The model under review builds one solid part; all positions refer to its coordinate system, in mm. A direction names the side the tool comes from. Give positions to 0.01 mm unless a question says otherwise; leave off trailing zeros. Order: outer loops, then holes, each group sorted by start corner. A loop starts at its lowest first (then second) coordinate and runs counter-clockwise, first axis right, second up. Notation, with made-up numbers: (-32, 2.5) -> (15, 2.5) arc R17 cw to (15, 6.5) -> close; hole circle Ø4 at (31, 37). An arc over 180 degrees is marked (long way). Answer as a JSON object with one key per item and string values. Group by question number.
Autodesk Inventor part; units mm, degrees
ref_plane "YZ Plane" through (0, 0, 0) normal (1, 0, 0) x (0, 1, 0)
ref_plane "XZ Plane" through (0, 0, 0) normal (0, 1, 0) x (-1, 0, 0)
ref_plane "XY Plane" through (0, 0, 0) normal (0, 0, 1) x (1, 0, 0)
sketch "Sketch1" plane through (0, 0, 0) normal (0, 0, 1) x (1, 0, 0)
  line L0 (-67, 0) -> (-70, 0)
  line L1 (-70, 0) -> (-70, 1)
  line L2 (-70, 1) -> (-67, 1)
  line L3 (-67, 1) -> (-67, 0)
  line L4 (-67, 0) -> (-69, 0)
  line L5 (-69, 0) -> (-69, -5)
  line L6 (-69, -5) -> (-67, -5)
  line L7 (-67, -5) -> (-67, 0)
  line L8 (-61.5, -0.5) -> (-67.5, -0.5)
  line L9 (-67.5, -0.5) -> (-67.5, -3)
  line L10 (-67.5, -3) -> (-61.5, -3)
  line L11 (-61.5, -3) -> (-61.5, -0.5)
  line L12 (-67, -3.5) -> (-68, -2.5)
  line L13 (-68, -2.5) -> (-68, -1)
  line L14 (-68, -1) -> (-67, 0)
  line L15 (0, -6.2) -> (0, 2.2)
  point P0 (0, 0)
  point P1 (-69, 0)
  point P2 (-67.5, -1.75)
  point P3 (-70, 0.5)
  point P4 (-68, -1.75)
  dimension "d0" = 5
  dimension "d1" = 69
  dimension "d4" = 1
  dimension "d5" = 2.5
  dimension "d6" = 67.5
  dimension "d7" = 67
  dimension "d9" = 3.5
  dimension "d11" = 2
  dimension "d12" = 6
  dimension "d13" = 0.5
  dimension "d27" = 0.5
  dimension "d28" = 1
revolve "Revolution1" add sketch "Sketch1" angle 360 about axis through (0, -10, 0) along (0, 1, 0) contours L14 L13 L12 L7 L6 L5 L0 | L0 L1 L2 L3
sketch "Sketch2" plane through (0, 1, 0) normal (0, 1, 0) x (1, 0, 0)
  circle A0 centre (-72.25, 0) radius 2.55
  point P0 (0, 0)
  dimension "d16" = 5.1
  dimension "d17" = 72.25
extrude "Extrusion1" cut sketch "Sketch2" against normal through all
sketch "Sketch3" plane through (0, -5, 0) normal (0, -1, 0) x (0, 0, 1)
  arc A0 (-68.9899, -1.1809) -> (-68.9899, 1.1809) centre (-71.25, 0) ccw
  circle A1 centre (-71.25, 0) radius 4
  point P0 (0, 0)
  dimension "d20" = 8
extrude "Extrusion2" [suppressed]
fillet "Fillet1" radius 4 2 edges at (-69.99, 0.5, -1.1811) (-69.99, 0.5, 1.1811)
pattern_circular "Circular Pattern1" [suppressed]
properties part number "Ring Bearing Track"
1. Machinability: for faces 4 (the flat face through (-52, 0, -46)), 5 (the cylindrical face through (-36.556, -1.74, 57.338)), 6 (the cylindrical face through (69.934, 0.507, 3.05)), which of the approach directions +Z, -Z, +X, -X, +Y, -Y give a long, thin tool a straight path to every point of the face, cutting with its end or side? Answer none if there is none.
2. Draft analysis for pull direction X (two halves, no side actions). For faces 1 (the flat face through (36, -5, 57)), 2 (the cylindrical face through (-65.814, -2.535, -20.726)), 3 (the cylindrical face through (14.524, -4.24, -65.407)), state which applies: pulls with the +X half, pulls with the -X half, needs draft (parallel to the pull), parting line crosses it, or undercut.
3. Take a section at A-A on x = 0. Give the boundary of the cut face in (y, z).
4. For pin 1 (1.5 mm diameter, centred on y = 0.5, z = -11.5, fed in from +X); pin 2 (3 mm diameter, centred on y = -1, z = 43, fed in from -X); pin 3 (2 mm diameter, centred on y = -2.5, z = 45, fed in from -X), all flat-tipped, find the tip position at first contact; note any pin that passes through.
5. For probe 1 along Z at (x, y) = (0, -1.7); probe 2 along Y at (x, z) = (64, 28); probe 3 along X at (y, z) = (0.5, -17.5), list the stretches that pass through material, from the lowest coordinate up. Write a range as [from, to].
Checks:
{
 "1": {"face 4": "-Y", "face 5": "none", "face 6": "+Y, -Y"},
 "2": {"face 1": "needs draft", "face 2": "parting line crosses it", "face 3": "undercut"},
 "3": {"outline": "(-5, -69) -> (0, -69) -> (0, -70) -> (1, -70) -> (1, -67) -> (0, -67) -> (-1, -68) -> (-2.5, -68) -> (-3.5, -67) -> (-5, -67) -> close; (-5, 67) -> (-3.5, 67) -> (-2.5, 68) -> (-1, 68) -> (0, 67) -> (1, 67) -> (1, 70) -> (0, 70) -> (0, 69) -> (-5, 69) -> close"},
 "4": {"pin 1": "stops at x = 69.17", "pin 2": "stops at x = -56.09", "pin 3": "stops at x = -53.15"},
 "5": {"probe 1": "z = [-69, -68], [68, 69]", "probe 2": "y = [0, 1]", "probe 3": "x = [-67.78, -64.67], [64.67, 67.78]"}
}
